Input: part model. Units: mm. Frame: model coordinates. Face numbers are marked on the shaded views. A direction names the side the tool comes from. Round coordinates to 2 decimals unless told otherwise and drop trailing zeros. Write each loop counter-clockwise with the first axis right and the second up, starting at its lowest first coordinate (ties: lowest second). Pieces come first, ordered by that corner, then holes. Notation, with made-up numbers: M 0,30.25 L 15,30.25 A25 cw 15,62.25 Z; hole C 71.5,40 d5. An arc over 180 degrees is marked long. Use one line per item in the form item = value. Start each with the question number.
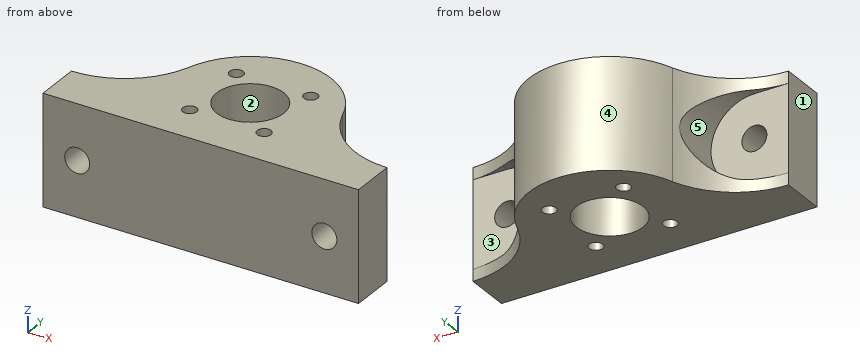
```python
from build123d import *

# Parameters (mm, degrees)
CROQUIS2_R              = 5.1
SALIENTE_EXTRUIR1_DEPTH = 16.8
CROQUIS3_R              = 1.05
CORTAR_EXTRUIR1_DEPTH   = 35.073450075
CORTAR_EXTRUIR2_DEPTH   = 35.073450075
CROQUIS5_R              = 1.9
CORTAR_EXTRUIR3_DEPTH   = 35.073450195


with BuildPart() as part:
    # Croquis2 → Saliente-Extruir1 (new body)
    with BuildSketch(Plane.XY):
        with BuildLine():
            Line((24, 0), (24, -6.9))
            Line((24, -6.9), (-24, -6.9))
            Line((-24, -6.9), (-24, 0))
            ThreePointArc((-24, 0), (-16.512763431, 2.381234531), (-11.776565713, 8.65))
            ThreePointArc((-11.776565713, 8.65), (0, 17.4), (11.776565713, 8.65))
            ThreePointArc((11.776565713, 8.65), (16.512763431, 2.381234531), (24, 0))
        make_face()
        with Locations((0, 5.1)):
            Circle(CROQUIS2_R, mode=Mode.SUBTRACT)
    extrude(amount=SALIENTE_EXTRUIR1_DEPTH)

    # Croquis3 → Cortar-Extruir1 (cut, through all)
    with BuildSketch(Plane.XY.offset(16.8)):
        with Locations((5.656854249, 10.756854249)):
            Circle(CROQUIS3_R)
        with Locations((5.656854249, -0.556854249)):
            Circle(CROQUIS3_R)
        with Locations((-5.656854249, -0.556854249)):
            Circle(CROQUIS3_R)
        with Locations((-5.656854249, 10.756854249)):
            Circle(CROQUIS3_R)
    extrude(amount=-CORTAR_EXTRUIR1_DEPTH, mode=Mode.SUBTRACT)

    # Croquis4 → Cortar-Extruir2 (cut, through all)
    with BuildSketch(Plane(origin=(0, 0, 0), x_dir=(1, 0, 0), z_dir=(0, 1, 0))):
        with BuildLine():
            Line((-24, -1.8), (-24, -15))
            Line((-24, -15), (-18.8, -15))
            ThreePointArc((-18.8, -15), (-12.2, -8.4), (-18.8, -1.8))
            Line((-18.8, -1.8), (-24, -1.8))
        make_face()
        with BuildLine():
            Line((24, -15), (18.8, -15))
            ThreePointArc((18.8, -15), (12.2, -8.4), (18.8, -1.8))
            Line((18.8, -1.8), (24, -1.8))
            Line((24, -1.8), (24, -15))
        make_face()
    extrude(amount=CORTAR_EXTRUIR2_DEPTH, mode=Mode.SUBTRACT)

    # Croquis5 → Cortar-Extruir3 (cut, through all)
    with BuildSketch(Plane(origin=(0, 0, 0), x_dir=(1, 0, 0), z_dir=(0, 1, 0))):
        with Locations(Location((-18.8, -8.4, 0), (0, 0, 270))):
            Circle(CROQUIS5_R)
        with Locations(Location((18.8, -8.4, 0), (0, 0, 270))):
            Circle(CROQUIS5_R)
    extrude(amount=-CORTAR_EXTRUIR3_DEPTH, mode=Mode.SUBTRACT)


solid = part.part
```
Item 1: Cut plane D-D (z = 8.4). Output: boundary loops of the cut face in (x, y).
Item 2: First-contact query: pin 1 (6 mm diameter, centred on x = -15.5, z = 9, fed in from +Y); pin 2 (1 mm diameter, centred on y = 2.5, z = 4.5, fed in from +X); pin 3 (1.5 mm diameter, centred on y = 11.5, z = 6, fed in from -X). Flat tips, straight axial feed; report the tip coordinate or a pass-through.
Item 3: Cut plane C-C (y = 5.1). Output: boundary loops of the cut face in (x, z).
Item 4: Cut plane B-B (z = 15.5). Output: boundary loops of the cut face in (x, y), plus the area to 3 significant figures.
Item 5: Reachability of the marked faces 4 and 5 from +Z, -Z, +X, -X, +Y, -Y: full face, straight path, thin tool, end or side. Return the list, or none.
Item 6: Draft query along X for the marked faces 1, 2 and 3. Return one class per face: +X half, -X half, draft (parallel to the pull), parting line (faces both ways), or undercut.
Item 7: Cut plane A-A (x = 0). Output: boundary loops of the cut face in (y, z), plus the area to 3 significant figures.
Item 8: Ray query, line 1 (Y direction, x = 19, z = 4.25); line 2 (Z direction, x = 15, y = 3.5); line 3 (Y direction, x = -3.5, z = 13.75). Return the intervals inside material, ascending. Write a range as from..to.
Final values:
q1.outline = M -24,-6.9 L -20.7,-6.9 L -20.7,0 L -24,0 Z; M -16.9,-6.9 L 16.9,-6.9 L 16.9,0 L 12.2,0 L 12.2,7.6 A12.96 cw 11.78,8.65 A12.3 ccw -11.78,8.65 A12.96 cw -12.2,7.6 L -12.2,0 L -16.9,0 Z; M 20.7,-6.9 L 24,-6.9 L 24,0 L 20.7,0 Z; hole C -5.66,-0.56 d2.1; hole C -5.66,10.76 d2.1; hole C 0,5.1 d10.2; hole C 5.66,-0.56 d2.1; hole C 5.66,10.76 d2.1
q2.pin_1 = 0
q2.pin_2 = 13.88
q2.pin_3 = -10.93
q3.outline = M -13.69,0 L -5.1,0 L -5.1,16.8 L -13.69,16.8 L -13.69,12.58 A6.6 cw -13.69,4.22 Z; M 5.1,0 L 13.69,0 L 13.69,4.22 A6.6 cw 13.69,12.58 L 13.69,16.8 L 5.1,16.8 Z
q4.outline = M -24,-6.9 L 24,-6.9 L 24,0 A12.96 cw 11.78,8.65 A12.3 ccw -11.78,8.65 A12.96 cw -24,0 Z; hole C -5.66,-0.56 d2.1; hole C -5.66,10.76 d2.1; hole C 0,5.1 d10.2; hole C 5.66,-0.56 d2.1; hole C 5.66,10.76 d2.1
q4.area = 648 mm^2
q5.face_4 = +Z, -Z, +Y
q5.face_5 = -X, +Y
q6.face_1 = -X half
q6.face_2 = undercut
q6.face_3 = draft
q7.outline = M -6.9,0 L 0,0 L 0,16.8 L -6.9,16.8 Z; M 10.2,0 L 17.4,0 L 17.4,16.8 L 10.2,16.8 Z
q7.area = 237 mm^2
q8.line_1 = -6.9..0
q8.line_2 = 0..3, 13.8..16.8
q8.line_3 = -6.9..1.39, 8.81..16.89
